Build history of the part. All positions in model axes, mm. Coordinates: 2 decimals unless noted, no trailing zeros. Write each loop counter-clockwise with the first axis right and the second up, starting at its lowest first coordinate (ties: lowest second). Pieces come first, ordered by that corner, then holes.
Autodesk Fusion 360 part; units mm, degrees
sketch "Sketch1" plane through (0, 0, 0) normal (0, 0, 1) x (1, 0, 0)
  line L0 (0, 0) -> (3, 0)
  line L1 (3, 0) -> (3, -20)
  line L2 (3, -20) -> (0, -20)
  line L3 (0, -20) -> (0, 0)
  line L4 (3, 0) -> (3.25, 0)
  line L5 (3.25, 0) -> (3.25, -20)
  line L6 (3.25, -20) -> (3, -20)
  line L7 (3, -20) -> (3, 0)
  line L8 (0, 0) -> (-0.25, 0)
  line L9 (-0.25, 0) -> (-0.25, -20)
  line L10 (-0.25, -20) -> (0, -20)
  line L11 (0, -20) -> (0, 0)
  line L12 (3.25, 0) -> (6.25, 0)
  line L13 (6.25, 0) -> (6.25, -20.0231)
  line L14 (6.25, -20.0231) -> (3.25, -20.0231)
  line L15 (3.25, -20.0231) -> (3.25, 0)
  line L16 (-0.25, 0) -> (-3.25, 0)
  line L17 (-3.25, 0) -> (-3.25, -20)
  line L18 (-3.25, -20) -> (-0.25, -20)
  line L19 (-0.25, -20) -> (-0.25, 0)
  dimension "d1" = 3
  dimension "d2" = 20
  dimension "d3" = 0.25
  dimension "d4" = 0.25
  dimension "d5" = 3
  dimension "d6" = 3
  dimension "d7" = 20
extrude "Extrude1" add sketch "Sketch1" along normal blind 3 contours L0 L1 L2 L3 L7 L11 | L3 L8 L9 L10 L11 L19 | L1 L4 L5 L6 L7 L15
extrude "Extrude2" add sketch "Sketch1" along normal blind 18 contours L9 L16 L17 L18 L19 | L5 L12 L13 L14 L15
extrude "Extrude3" add 1 faces at (5.25, -6.6744, 18) along direction (0, 0, 1) blind 15
extrude "Extrude4" cut 1 faces at (5.25, -6.6744, 33) along direction (0, 0, -1) blind 15
extrude "Extrude5" add 1 faces at (-2.25, 0, 7) along direction (0, 1, 0) blind 20
1. Saw through at B-B on y = 10. List the corners of the cut face in (x, z), plus the area to 4 significant figures.
Computed values:
outline: (-3.25, 0) - (6.25, 0) - (6.25, 18) - (3.25, 18) - (3.25, 3) - (-0.25, 3) - (-0.25, 18) - (-3.25, 18) - close
area: 118.5 mm2
2. Flat gauge pins, fed straight in: pin 1 (1.8 mm diameter, centred on x = 2, y = 5, fed in from +Z); pin 2 (3 mm diameter, centred on x = 0, y = 15.5, fed in from +Z). Where does each tip first touch, or does it go through?
Computed values:
pin 1: stops at z = 3
pin 2: stops at z = 18
3. Probe line 1 along X through (y, z) = (1.5, 14); line 2 along Z through (x, y) = (1.5, -9.5); line 3 along Y through (x, z) = (-2.5, 16.5). List the from-to ranges inside material, lowest first.
Computed values:
line 1: x = -3.25 to -0.25, 3.25 to 6.25
line 2: z = 0 to 3
line 3: y = -20 to 20
4. Saw through at A-A on z = 5.75. List the corners of the cut face in (x, y), plus the area to 3 significant figures.
Computed values:
outline: (-3.25, -20) - (-0.25, -20) - (-0.25, 20) - (-3.25, 20) - close; (3.25, -20.02) - (6.25, -20.02) - (6.25, 20) - (3.25, 20) - close
area: 240 mm2
5. Mould opens along X. For faces 1 (the face through (3.25, 0, 11)), 2 (the face through (-1, 20, 9)), 3 (the face through (1, 0, 3)), 4 (the face through (6.25, 0, 9)) say: +X half, -X half, draft (parallel to the pull), parting line (faces both ways), or undercut.
Computed values:
face 1: undercut
face 2: draft
face 3: undercut
face 4: +X half
6. Saw through at C-C on x = 1. List the corners of the cut face in (y, z), plus the area to 3 significant figures.
Computed values:
outline: (-20, 0) - (20, 0) - (20, 3) - (-20, 3) - close
area: 120 mm2
